Autodesk Inventor part; units mm, degrees
ref_plane "YZ Plane" through (0, 0, 0) normal (1, 0, 0) x (0, 1, 0)
ref_plane "XZ Plane" through (0, 0, 0) normal (0, 1, 0) x (-1, 0, 0)
ref_plane "XY Plane" through (0, 0, 0) normal (0, 0, 1) x (1, 0, 0)
sketch "Sketch1" plane through (0, 0, 0) normal (0, 0, 1) x (1, 0, 0)
  circle A0 centre (0, 0) radius 50
  arc A1 (-73.4116, 137.5742) -> (0, 87.1574) centre (-8.4976, 153.4397) ccw
  arc A2 (-73.4116, 137.5742) -> (-123.2383, 133.4142) centre (-96.0994, 108.8375) ccw
  arc A3 (-123.2383, 133.4142) -> (-105.1177, 55.113) centre (-61.0095, 106.5679) ccw
  arc A4 (-49.9992, -0.286) -> (-105.1177, 55.113) centre (-114.9857, -9.8243) ccw
  line L0 (-25, 0) -> (25, 0)
  line L1 (25, 0) -> (25, -100)
  line L2 (25, -100) -> (-25, -100)
  line L3 (-25, -100) -> (-25, 0)
  line L4 (0, 63.4714) -> (21.5005, 63.4714) construction
  line L5 (-99.5328, 106.1382) -> (-94.5328, 106.1382)
  line L6 (-94.5328, 106.1382) -> (-94.5328, 86.1382)
  line L7 (-94.5328, 86.1382) -> (-99.5328, 86.1382)
  line L8 (-99.5328, 86.1382) -> (-99.5328, 106.1382)
  arc A5 (0, 87.1574) -> (73.4116, 137.5742) centre (8.4976, 153.4397) ccw
  arc A6 (123.2383, 133.4142) -> (73.4116, 137.5742) centre (96.0994, 108.8375) ccw
  arc A7 (105.1177, 55.113) -> (123.2383, 133.4142) centre (61.0095, 106.5679) ccw
  arc A8 (105.1177, 55.113) -> (49.9992, -0.286) centre (114.9857, -9.8243) ccw
  line L9 (99.5328, 106.1382) -> (94.5328, 106.1382)
  line L10 (94.5328, 106.1382) -> (94.5328, 86.1382)
  line L11 (94.5328, 86.1382) -> (99.5328, 86.1382)
  line L12 (99.5328, 86.1382) -> (99.5328, 106.1382)
  line L13 (49.9992, -0.286) -> (-49.9992, -0.286)
  line L14 (-7.7212, -92.2433) -> (-3.7298, -89.2319)
  line L15 (-3.7298, -89.2319) -> (-15.7757, -73.2664)
  line L16 (-15.7757, -73.2664) -> (-19.7671, -76.2779)
  line L17 (-19.7671, -76.2779) -> (-7.7212, -92.2433)
  line L18 (7.7212, -92.2433) -> (3.7298, -89.2319)
  line L19 (3.7298, -89.2319) -> (15.7757, -73.2664)
  line L20 (15.7757, -73.2664) -> (19.7671, -76.2779)
  line L21 (19.7671, -76.2779) -> (7.7212, -92.2433)
  dimension "d0" = 100
  dimension "d4" = 50
  dimension "d5" = 50
  dimension "d6" = 100
  dimension "d8" = 5
  dimension "d9" = 20
  dimension "d10" = 5
  dimension "d11" = 20
  dimension "d12" = 5
extrude "Extrusion2" add sketch "Sketch1" along normal blind 5.5 contours A0 L13 L1 L0 L3 | A0 A4 A3 A2 A1 A5 A6 A7 A8 | L13 L3 A0 | A0 L1 L13 | L3 L13 L1 A0 | A0 L1 L2 L3 | L3 L0 L1 L13 | L17 L16 L15 L14 | L18 L19 L20 L21
fillet "Fillet4" radius 2 4 edges at (-99.5328, 106.1382, 2.75) (-94.5328, 106.1382, 2.75) (-94.5328, 86.1382, 2.75) (-99.5328, 86.1382, 2.75)
fillet "Fillet5" radius 2 4 edges at (99.5328, 86.1382, 2.75) (99.5328, 106.1382, 2.75) (94.5328, 106.1382, 2.75) (94.5328, 86.1382, 2.75)
sketch "Sketch2" plane through (0, 0, 5.5) normal (0, 0, 1) x (1, 0, 0)
  line L0 (-10, -80) -> (10, -80)
  line L1 (10, -80) -> (10, -75)
  line L2 (10, -75) -> (-10, -75)
  line L3 (-10, -75) -> (-10, -80)
  point P0 (0, 0)
  dimension "d20" = 20
  dimension "d21" = 5
extrude "Extrusion3" cut sketch "Sketch2" against normal blind 5.5
fillet "Fillet6" radius 5 2 edges at (25, -100, 2.75) (-25, -100, 2.75)
fillet "Fillet7" radius 2 4 edges at (-10, -75, 2.75) (-10, -80, 2.75) (10, -80, 2.75) (10, -75, 2.75)
fillet "Fillet8" radius 2 2 edges at (-105.1177, 55.113, 2.75) (105.1177, 55.113, 2.75)
sketch "Sketch4" plane through (0, 0, 5.5) normal (0, 0, 1) x (1, 0, 0)
  line L0 (30, 2.7) -> (-30, 2.7)
  line L1 (-30, 2.7) -> (-30, -2.7)
  line L2 (-30, -2.7) -> (30, -2.7)
  line L3 (30, -2.7) -> (30, 2.7)
  point P0 (0, 0)
  dimension "d34" = 60
  dimension "d35" = 5.4
extrude "Extrusion5" cut sketch "Sketch4" against normal blind 10
sketch "Sketch5" plane through (0, 0, 5.5) normal (0, 0, 1) x (1, 0, 0)
  line L0 (39.75, 2.75) -> (45.25, 2.75)
  line L1 (45.25, 2.75) -> (45.25, -2.75)
  line L2 (45.25, -2.75) -> (39.75, -2.75)
  line L3 (39.75, -2.75) -> (39.75, 2.75)
  line L4 (-39.75, -2.75) -> (-45.25, -2.75)
  line L5 (-45.25, -2.75) -> (-45.25, 2.75)
  line L6 (-45.25, 2.75) -> (-39.75, 2.75)
  line L7 (-39.75, 2.75) -> (-39.75, -2.75)
  point P0 (0, 0)
  point P1 (0, 0)
  dimension "d40" = 5.5
  dimension "d41" = 5.5
  dimension "d42" = 360
extrude "Extrusion6" cut sketch "Sketch5" against normal blind 10
properties part number "central"
Part model, mm, in its own coordinate system. A direction names the side the tool comes from. Round coordinates to 2 decimals unless told otherwise and drop trailing zeros. Loops run counter-clockwise (first coordinate to the right, second up) from the corner with the lowest first, then second, coordinate; pieces in that order, holes last.
Item 1: Drill centre lines: line 1 (X direction, y = -57, z = 3.5); line 2 (X direction, y = 125.5, z = 2.6); line 3 (Y direction, x = 22.5, z = 0.9). Where is each one in solid material? Low to high.
Item 2: Mould opens along Y. For faces 1 (the face through (42, 2.75, 3)), 2 (the face through (-99.53, 145.29, 2.71)), 3 (the face through (-2, 52, 0)) say: +Y half, -Y half, draft (parallel to the pull), parting line (faces both ways), or undercut.
Item 3: Cut at C-C, the plane y = -72. Give the cut face in (x, z).
Item 4: 3-axis set-ups, long thin cutter, end or side, ignore diameter. For faces 4 (the face through (25, -69, 3)), 5 (the face through (-126.967, 90.988, 2.712)), 6 (the face through (-45.25, 0, 3)): which of +Z, -Z, +X, -X, +Y, -Y reach the whole face in a straight line?
Item 5: Cut at B-B, the plane x = 13.5. Give the cut face in (y, z).
Item 6: Cut at A-A, the plane y = 130.5. Give the cut face in (x, z), then the cut area to 3 significant figures.
Item 7: Drop flat-ended pins along their axis: P1, Ø1.6, axis at y = 99, z = 3.5, coming from the -X side; P2, Ø4, axis at x = 42, y = 77, coming from the -Z side; P3, Ø3, axis at y = -40.5, z = 4, coming from the -X side; P4, Ø3, axis at x = 42.5, z = 2.5, coming from the +Y side. Give the stop position or say it passes through.
Item 8: Cut at D-D, the plane z = 2.55. State how many separate pieces and enclosed holes the cut face has, then the cut area to 3 significant figures.
A:
1. line 1: x = -25 to 25
1. line 2: x = -126.08 to -69.2, 69.2 to 126.08
1. line 3: y = -99.33 to -2.7, 2.7 to 88.1
2. face 1: undercut
2. face 2: +Y half
2. face 3: draft
3. outline: (-25, 0) - (25, 0) - (25, 5.5) - (-25, 5.5) - close
4. face 4: +Z, -Z, +X, -Y
4. face 5: +Z, -Z, -X
4. face 6: +Z, -Z
5. outline: (-100, 0) - (-2.7, 0) - (-2.7, 5.5) - (-100, 5.5) - close; (2.7, 0) - (86.8, 0) - (86.8, 5.5) - (2.7, 5.5) - close
6. outline: (-124.42, 0) - (-71.26, 0) - (-71.26, 5.5) - (-124.42, 5.5) - close; (71.26, 0) - (124.42, 0) - (124.42, 5.5) - (71.26, 5.5) - close
6. area: 585 mm2
7. P1: stops at x = -128.44
7. P2: stops at z = 0
7. P3: stops at x = -31.29
7. P4: stops at y = 96.83
8. separate pieces: 1
8. enclosed holes: 6
8. area: 28,100 mm2
